For this review, use the dimensioned drawing (mm, ordinates from the lowest corner) and the shaded views. A direction names the side the tool comes from. Give positions to 0.01 mm unless a question says otherwise; leave off trailing zeros. Order: outer loops, then holes, each group sorted by start corner. A loop starts at its lowest first (then second) coordinate and runs counter-clockwise, first axis right, second up.
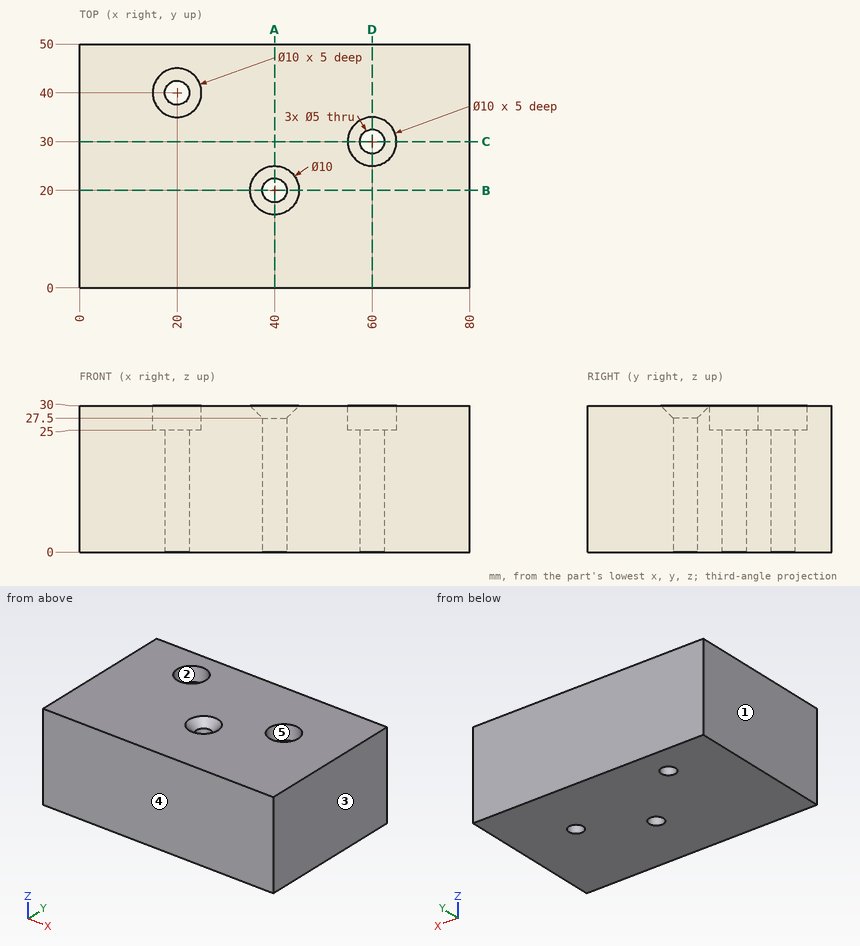
1. For the marked faces 1 and 2, list the 3-axis set-ups (+Z, -Z, +X, -X, +Y, -Y) from which the entire face can be reached by the end or side of a thin tool; tool diameter is ignored.
2. To check wall thickness, follow line 1 (Y direction, x = 60, z = 26.2); line 2 (Y direction, x = 40, z = 21.5); line 3 (Z direction, x = 22, y = 44.5). State the ranges of each line that lie inside material, in increasing order.
3. Take a section at A-A (x = 40). Write out the cut boundary in (y, z), and give its area (3 significant figures).
4. Take a section at C-C (y = 30). Write out the cut boundary in (x, z), and give its area (4 significant figures).
5. Draft analysis for pull direction Y (two halves, no side actions). For the marked faces 3, 4 and 5, state which applies: pulls with the +Y half, pulls with the -Y half, needs draft (parallel to the pull), parting line crosses it, or undercut.
6. Insertion check: pin 1 (6 mm diameter, centred on x = 20, y = 40, fed in from +Z). The pin has a flat end and moves straight along its axis. Give the tip position at first contact, or say it passes through.
7. Take a section at D-D (x = 60). Write out the cut boundary in (y, z), and give its area (4 significant figures).
8. Take a section at B-B (y = 20). Write out the cut boundary in (x, z).
Answer:
1. face 1: +Z, -Z, -X, +Y, -Y
1. face 2: +Z
2. line 1: y = 0 to 25, 35 to 50
2. line 2: y = 0 to 17.5, 22.5 to 50
2. line 3: z = 0 to 25
3. outline: (0, 0) - (17.5, 0) - (17.5, 27.5) - (15, 30) - (0, 30) - close; (22.5, 0) - (50, 0) - (50, 30) - (25, 30) - (22.5, 27.5) - close
3. area: 1,340 mm2
4. outline: (0, 0) - (57.5, 0) - (57.5, 25) - (55, 25) - (55, 30) - (0, 30) - close; (62.5, 0) - (80, 0) - (80, 30) - (65, 30) - (65, 25) - (62.5, 25) - close
4. area: 2,225 mm2
5. face 3: needs draft
5. face 4: pulls with the -Y half
5. face 5: undercut
6. pin 1: stops at z = 25
7. outline: (0, 0) - (27.5, 0) - (27.5, 25) - (25, 25) - (25, 30) - (0, 30) - close; (32.5, 0) - (50, 0) - (50, 30) - (35, 30) - (35, 25) - (32.5, 25) - close
7. area: 1,325 mm2
8. outline: (0, 0) - (37.5, 0) - (37.5, 27.5) - (35, 30) - (0, 30) - close; (42.5, 0) - (80, 0) - (80, 30) - (45, 30) - (42.5, 27.5) - close
